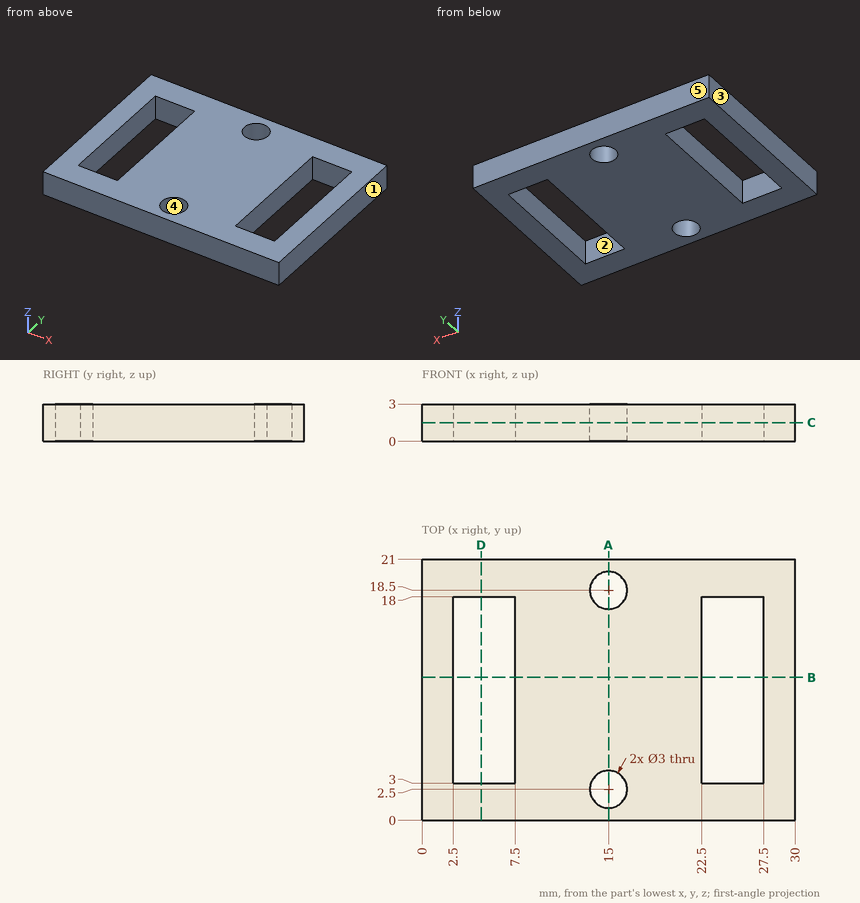
Study the drawing (mm; zero at the part's minimum x, y, z) and answer. A direction names the side the tool comes from. Give positions to 0.01 mm unless a question says otherwise; leave off trailing zeros. Write each loop counter-clockwise with the first axis right and the second up, starting at its lowest first coordinate (ties: lowest second). Pieces come first, ordered by that corner, then holes. Notation, with made-up numbers: (-22, 26) - (-11, 26) arc R28 ccw to (-11, 56) - close; hole circle Ø1 at (54.25, 80.25). An arc over 180 degrees is marked (long way). One line per question, with ' | ' between items. Start each with the question number.
1. Section D-D, the plane x = 4.75 is taken. Determine the outline of the cut face in (y, z).
2. Section B-B, the plane y = 11.5 is taken. Determine the outline of the cut face in (x, z), then the cut area to 3 significant figures.
3. Given P1, Ø2.5, axis at x = 15, y = 18.5, coming from the +Z side, flat-ended and moving along its own axis, determine where the tip first touches the part or whether it passes through.
4. Determine the mould class of the marked faces 3, 4 and 5 for opening direction Y: +Y half, -Y half, draft (parallel to the pull), parting line (faces both ways), or undercut.
5. Straight lines are drawn through the part: line 1 (X direction, y = 7.5, z = 2); line 2 (Y direction, x = 15, z = 1.9); line 3 (X direction, y = 2.5, z = 2.15). For each, find the intervals that lie inside material, in ascending order.
6. Section C-C, the plane z = 1.5 is taken. Determine the outline of the cut face in (x, y).
7. Section A-A, the plane x = 15 is taken. Determine the outline of the cut face in (y, z).
8. For the marked faces 1 and 2, determine the directions among +Z, -Z, +X, -X, +Y, -Y from which every point of the face is accessible in a straight line to the end or side of a thin tool.
Result:
1) outline: (0, 0) - (3, 0) - (3, 3) - (0, 3) - close; (18, 0) - (21, 0) - (21, 3) - (18, 3) - close
2) outline: (0, 0) - (2.5, 0) - (2.5, 3) - (0, 3) - close; (7.5, 0) - (22.5, 0) - (22.5, 3) - (7.5, 3) - close; (27.5, 0) - (30, 0) - (30, 3) - (27.5, 3) - close | area: 60.0 mm2
3) P1: passes through
4) face 3: draft | face 4: undercut | face 5: +Y half
5) line 1: x = 0 to 2.5, 7.5 to 22.5, 27.5 to 30 | line 2: y = 0 to 1, 4 to 17, 20 to 21 | line 3: x = 0 to 13.5, 16.5 to 30
6) outline: (0, 0) - (30, 0) - (30, 21) - (0, 21) - close; hole (2.5, 3) - (7.5, 3) - (7.5, 18) - (2.5, 18) - close; hole circle Ø3 at (15, 2.5); hole circle Ø3 at (15, 18.5); hole (22.5, 3) - (27.5, 3) - (27.5, 18) - (22.5, 18) - close
7) outline: (0, 0) - (1, 0) - (1, 3) - (0, 3) - close; (4, 0) - (17, 0) - (17, 3) - (4, 3) - close; (20, 0) - (21, 0) - (21, 3) - (20, 3) - close
8) face 1: +Z, -Z, +X, +Y, -Y | face 2: +Z, -Z
